Autodesk Inventor part; units mm, degrees
ref_plane "YZ Plane" through (0, 0, 0) normal (1, 0, 0) x (0, 1, 0)
ref_plane "XZ Plane" through (0, 0, 0) normal (0, 1, 0) x (-1, 0, 0)
ref_plane "XY Plane" through (0, 0, 0) normal (0, 0, 1) x (1, 0, 0)
sketch "Face" plane through (0, 0, 0) normal (0, 0, 1) x (1, 0, 0)
  circle A0 centre (143.9602, -80.6846) radius 6.35
  circle A1 centre (39.7975, -186.0352) radius 2.4
  circle A2 centre (85.2205, -107.3602) radius 2.4
  circle A3 centre (130.6435, -186.0352) radius 2.4
  circle A4 centre (85.2205, -159.8102) radius 42.45
  circle A5 centre (14.75, -202.58) radius 2.6
  circle A6 centre (165.25, -202.58) radius 2.6
  circle A7 centre (14.75, -40.38) radius 2.6
  circle A8 centre (165.25, -40.38) radius 2.6
  line L0 (180, 0) -> (0, 0)
  line L1 (0, 0) -> (0, -250)
  line L2 (0, -250) -> (180, -250)
  line L3 (180, -250) -> (180, 0)
  point P0 (94.9979, -134.0949)
  point P1 (175.25, -245.25)
sketch "Sketch1" plane through (0, 0, 0) normal (1, 0, 0) x (0, 1, 0)
  circle A0 centre (53.9602, 44.3154) radius 6.35
  circle A1 centre (-50.2025, -61.0352) radius 2.4
  circle A2 centre (-4.7795, 17.6398) radius 2.4
  circle A3 centre (40.6435, -61.0352) radius 2.4
  circle A4 centre (-4.7795, -34.8102) radius 42.45
  circle A5 centre (-75.25, -77.58) radius 2.6
  circle A6 centre (75.25, -77.58) radius 2.6
  circle A7 centre (-75.25, 84.62) radius 2.6
  circle A8 centre (75.25, 84.62) radius 2.6
  line L0 (90, 125) -> (-90, 125)
  line L1 (-90, 125) -> (-90, -125)
  line L2 (-90, -125) -> (90, -125)
  line L3 (90, -125) -> (90, 125)
  point P0 (0, 0)
  point P1 (-90, 0)
  point P2 (0, 125)
extrude "Extrusion1" add sketch "Sketch1" along normal mid plane 4.75 contours A0 | L3 L2 L1 L0
sketch "Sketch2" plane through (2.375, 0, 0) normal (1, 0, 0) x (0, 0, -1)
  circle A0 centre (-17.6398, -4.7795) radius 2.4
  circle A1 centre (61.0352, -50.2025) radius 2.4
  circle A2 centre (61.0352, 40.6435) radius 2.4
  point P0 (0, 0)
hole "Hole1" at (2.375, -4.7795, 17.6398) at (2.375, -50.2025, -61.0352) at (2.375, 40.6435, -61.0352) direction (-1, 0, 0) diameter 5.5 end through all
properties part number "BREEZE-M08"
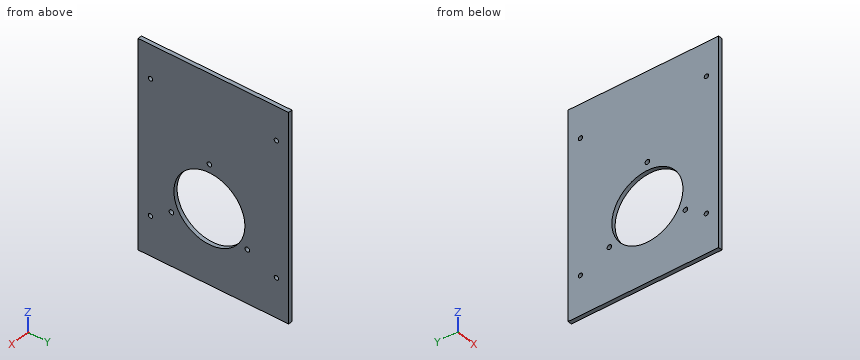
Here's how the part is built. I have some questions about the finished solid (model axes, mm). Coordinates: 2 decimals unless noted, no trailing zeros. Order: outer loops, then holes, each group sorted by start corner. A loop starts at its lowest first (then second) coordinate and runs counter-clockwise, first axis right, second up.
1) Imagine slicing it at B-B on y = 75.25. List the corners of the cut face in (x, z) for me (3 decimals).
2) Will this pin go through, and if not, where does the flat tip stop? pin 1 (4 mm diameter, centred on y = -75.25, z = 84.62, fed in from -X).
3) Imagine slicing it at A-A on z = 84.62. List the corners of the cut face in (x, y) for me (3 decimals).
4) Imagine slicing it at D-D on z = -10. List the corners of the cut face in (x, y) for me (3 decimals), and give its area (3 significant figures).
5) Imagine slicing it at C-C on y = -26. List the corners of the cut face in (x, z) for me (3 decimals), and give its area (3 significant figures).
6) I need wall thicknesses on line 1 (Z direction, x = 1.1, y = -75.25); line 2 (Z direction, x = -1.05, y = -76.5); line 3 (Z direction, x = -1.55, y = 42.5). Which ranges of each line are inside material? Lowest first, please.
Response values:
1. outline: (-2.375, -125) - (2.375, -125) - (2.375, -80.18) - (-2.375, -80.18) - close; (-2.375, -74.98) - (2.375, -74.98) - (2.375, 82.02) - (-2.375, 82.02) - close; (-2.375, 87.22) - (2.375, 87.22) - (2.375, 125) - (-2.375, 125) - close
2. pin 1: passes through
3. outline: (-2.375, -90) - (2.375, -90) - (2.375, -77.85) - (-2.375, -77.85) - close; (-2.375, -72.65) - (2.375, -72.65) - (2.375, 72.65) - (-2.375, 72.65) - close; (-2.375, 77.85) - (2.375, 77.85) - (2.375, 90) - (-2.375, 90) - close
4. outline: (-2.375, -90) - (2.375, -90) - (2.375, -39.224) - (-2.375, -39.224) - close; (-2.375, 29.665) - (2.375, 29.665) - (2.375, 90) - (-2.375, 90) - close
4. area: 528 mm2
5. outline: (-2.375, -125) - (2.375, -125) - (2.375, -71.576) - (-2.375, -71.576) - close; (-2.375, 1.955) - (2.375, 1.955) - (2.375, 125) - (-2.375, 125) - close
5. area: 838 mm2
6. line 1: z = -125 to -80.18, -74.98 to 82.02, 87.22 to 125
6. line 2: z = -125 to -79.86, -75.3 to 82.34, 86.9 to 125
6. line 3: z = -125 to -63.06, -59.01 to 125
